Here's how the part is built. I have some questions about the finished solid (model axes, mm). Give positions to 0.01 mm unless a question says otherwise; leave off trailing zeros. Loops run counter-clockwise (first coordinate to the right, second up) from the corner with the lowest first, then second, coordinate; pieces in that order, holes last.
Q1. If we section it at B-B (z = 15): Please give me the cut outline in (x, y).
Q2. I need wall thicknesses on line 1 (X direction, y = -0.3, z = 15); line 2 (X direction, y = -0.25, z = 14); line 3 (Z direction, x = -3, y = -0.15). Which ranges of each line are inside material? Lowest first, please.
Q3. We'd pull the mould along Z, two halves only. Please class faces 1 (the face through (1.05, -0.25, 18.34)), 2 (the face through (-2, 0, 0)): +Z half, -Z half, draft (parallel to the pull), parting line (faces both ways), or undercut.
Q4. If we section it at A-A (x = 0): Please give me the cut outline in (y, z).
from build123d import *

# Parameters (mm, degrees)
SKETCH1_W            = 245
SKETCH1_H            = 50
BASE_FLANGE1_DEPTH   = 0.5
SKETCH6_R            = 3.5
CUT_EXTRUDE1_DEPTH   = 10
LPATTERN1_COUNT      = 6
LPATTERN1_PITCH      = 146
LPATTERN1_COUNT_DIR2 = 6
LPATTERN1_PITCH_DIR2 = 146
LPATTERN2_COUNT      = 2
LPATTERN2_PITCH      = 100
LPATTERN2_COL_COUNT  = 2
LPATTERN2_COL_PITCH  = 100


# Sheet-metal steps are written as plain solids
with BuildPart() as part:
    # Sketch1 → Base-Flange1 (new body)
    with BuildSketch(Plane(origin=(0, 0, 0), x_dir=(1, 0, 0), z_dir=(0, 1, 0))):
        Rectangle(SKETCH1_W, SKETCH1_H)
    extrude(amount=-BASE_FLANGE1_DEPTH)

    # Sketch6 → Cut-Extrude1 (cut)
    with BuildSketch(Plane(origin=(0, 0, 0), x_dir=(1, 0, 0), z_dir=(0, 1, 0))):
        with Locations(Location((0, -15, 0), (0, 0, 270))):
            Circle(SKETCH6_R)
    cut_extrude1 = extrude(amount=-CUT_EXTRUDE1_DEPTH, mode=Mode.SUBTRACT)

    # LPattern1: Cut-Extrude1 6 × 6
    with Locations(*[Vector(-1, 0, 0) * (i * LPATTERN1_PITCH) + Vector(1, 0, 0) * (j * LPATTERN1_PITCH_DIR2) for i in range(LPATTERN1_COUNT) for j in range(LPATTERN1_COUNT_DIR2) if (i, j) != (0, 0)]):
        add(cut_extrude1, mode=Mode.SUBTRACT)

    # LPattern2: Cut-Extrude1 ×2
    with Locations(*[(-i * LPATTERN2_PITCH, 0, 0) for i in range(1, LPATTERN2_COUNT)]):
        add(cut_extrude1, mode=Mode.SUBTRACT)

    # LPattern2 col: Cut-Extrude1 ×2
    with Locations(*[(i * LPATTERN2_COL_PITCH, 0, 0) for i in range(1, LPATTERN2_COL_COUNT)]):
        add(cut_extrude1, mode=Mode.SUBTRACT)


solid = part.part
Check sheet entries:
1. outline: (-122.5, -0.5) - (-103.5, -0.5) - (-103.5, 0) - (-122.5, 0) - close; (-96.5, -0.5) - (-3.5, -0.5) - (-3.5, 0) - (-96.5, 0) - close; (3.5, -0.5) - (96.5, -0.5) - (96.5, 0) - (3.5, 0) - close; (103.5, -0.5) - (122.5, -0.5) - (122.5, 0) - (103.5, 0) - close
2. line 1: x = -122.5 to -103.5, -96.5 to -3.5, 3.5 to 96.5, 103.5 to 122.5
2. line 2: x = -122.5 to -103.35, -96.65 to -3.35, 3.35 to 96.65, 103.35 to 122.5
2. line 3: z = -25 to 13.2, 16.8 to 25
3. face 1: undercut
3. face 2: draft
4. outline: (-0.5, -25) - (0, -25) - (0, 11.5) - (-0.5, 11.5) - close; (-0.5, 18.5) - (0, 18.5) - (0, 25) - (-0.5, 25) - close
